Work out the finished part from the listing and answer in its coordinate system (mm). A direction names the side the tool comes from. Coordinates: 2 decimals unless noted, no trailing zeros. Loops run counter-clockwise (first coordinate to the right, second up) from the corner with the lowest first, then second, coordinate; pieces in that order, holes last. Notation, with made-up numbers: (68, 27.5) - (87, 27.5) arc R13 cw to (87, 49.5) - close; hole circle Ø9 at (32, 63). An arc over 180 degrees is marked (long way). Write each question's results on one line, items separated by ' | '. Start each with the question number.
1. Find the intervals of material crossed by line 1 along Z through (x, y) = (692, -0.2); line 2 along Z through (x, y) = (714.5, -0.4); line 3 along X through (y, z) = (-1.3, -566), in increasing order. Write a range as [from, to].
2. Which of the six approach directions +Z, -Z, +X, -X, +Y, -Y give full straight-line access (tool end or side, diameter ignored) to faces 1 (the flat face through (763, 0, -518)), 2 (the flat face through (659.62, -1.69, -539.42))?
3. Determine the mould class of faces 3 (the cylindrical face through (855.795, -1.69, -572.932)), 4 (the flat face through (763, -3.429, -518)), 5 (the flat face through (881.686, -1.69, -497.421)) for opening direction Z: released by +Z, released by -Z, zero draft, split by the parting line, or undercut.
4. A cutting plane is placed at D-D on z = -512.5. Determine the outline of the cut face in (x, y), then the cut area to 3 significant figures.
5. A cutting plane is placed at C-C on z = -568.5. Determine the outline of the cut face in (x, y).
6. A cutting plane is placed at A-A on y = -1.9. Determine the outline of the cut face in (x, z).
7. A cutting plane is placed at B-B on x = 692. Determine the outline of the cut face in (y, z).
8. Each of these flat-tipped pins is pushed along its axis until it touches: P1, Ø1.6, axis at y = -1, z = -492.5, coming from the +X side; P2, Ø1.7, axis at x = 688.5, y = -2, coming from the +Z side; P3, Ø1, axis at y = -1.5, z = -552, coming from the -X side. Where does it stop, or does it pass through?
from build123d import *

# Parameters (mm, degrees)
F1_DEPTH = 3.429


# Not quite as in the source:
# - ends of sketch curves that miss each other by under 0.0002 mm in the source are joined


with BuildPart() as f1:
    # F0 (on Front) → F1 (new body)
    with BuildSketch(Plane.XZ):
        Polygon((718.4461374, -491.0265008), (700.6661374, -491.0265008), (700.6661374, -494.2015008), (668.9161374, -494.2015008), (629.8223878, -533.2952504), (627.5773072, -531.0501952), (615.0049422, -543.6225348), (617.2500228, -545.8676154), (578.1562732, -584.961365), (578.1562732, -589.4515008), (884.8161374, -589.4515008), (884.8161374, -500.5515008), (878.4661374, -494.2015008), (853.0661374, -494.2015008), (853.0661374, -491.0265008), (835.2861374, -491.0265008), (835.2861374, -494.2015008), (718.4461374, -494.2015008), align=None)
        with BuildLine():
            ThreePointArc((859.4161374, -564.0515008), (855.6963935211, -573.0317569211), (846.7161374, -576.7515008))
            Line((846.7161374, -576.7515008), (652.9476654, -576.7515008))
            ThreePointArc((652.9476654, -576.7515008), (641.2143919005, -568.9115720944), (643.9674219789, -555.0712319789))
            Line((643.9674219789, -555.0712319789), (675.7174192, -523.3212292))
            ThreePointArc((675.7174192, -523.3212292), (679.8375941056, -520.5682273005), (684.6976654, -519.6015008))
            Line((684.6976654, -519.6015008), (846.7161374, -519.6015008))
            ThreePointArc((846.7161374, -519.6015008), (855.6963935211, -523.3212446789), (859.4161374, -532.3015008))
            Line((859.4161374, -532.3015008), (859.4161374, -564.0515008))
        make_face(mode=Mode.SUBTRACT)
    extrude(amount=F1_DEPTH)


solid = f1.part
Values:
1) line 1: [-589.45, -576.75], [-519.6, -494.2] | line 2: [-589.45, -576.75], [-519.6, -491.03] | line 3: [597.12, 640.4], [859.27, 884.82]
2) face 1: +Z, -Z, +X, -X, +Y | face 2: +Y, -Y
3) face 3: undercut | face 4: zero draft | face 5: released by +Z
4) outline: (650.62, -3.43) - (884.82, -3.43) - (884.82, 0) - (650.62, 0) - close | area: 803 mm^2
5) outline: (594.62, -3.43) - (641.05, -3.43) - (641.05, 0) - (594.62, 0) - close; (858.61, -3.43) - (884.82, -3.43) - (884.82, 0) - (858.61, 0) - close
6) outline: (578.16, -589.45) - (884.82, -589.45) - (884.82, -500.55) - (878.47, -494.2) - (853.07, -494.2) - (853.07, -491.03) - (835.29, -491.03) - (835.29, -494.2) - (718.45, -494.2) - (718.45, -491.03) - (700.67, -491.03) - (700.67, -494.2) - (668.92, -494.2) - (629.82, -533.3) - (627.58, -531.05) - (615, -543.62) - (617.25, -545.87) - (578.16, -584.96) - close; hole (643.97, -555.07) arc R12.7 ccw to (652.95, -576.75) - (846.72, -576.75) arc R12.7 ccw to (859.42, -564.05) - (859.42, -532.3) arc R12.7 ccw to (846.72, -519.6) - (684.7, -519.6) arc R12.7 ccw to (675.72, -523.32) - close
7) outline: (-3.43, -589.45) - (0, -589.45) - (0, -576.75) - (-3.43, -576.75) - close; (-3.43, -519.6) - (0, -519.6) - (0, -494.2) - (-3.43, -494.2) - close
8) P1: x = 853.07 | P2: z = -494.2 | P3: x = 610.62
